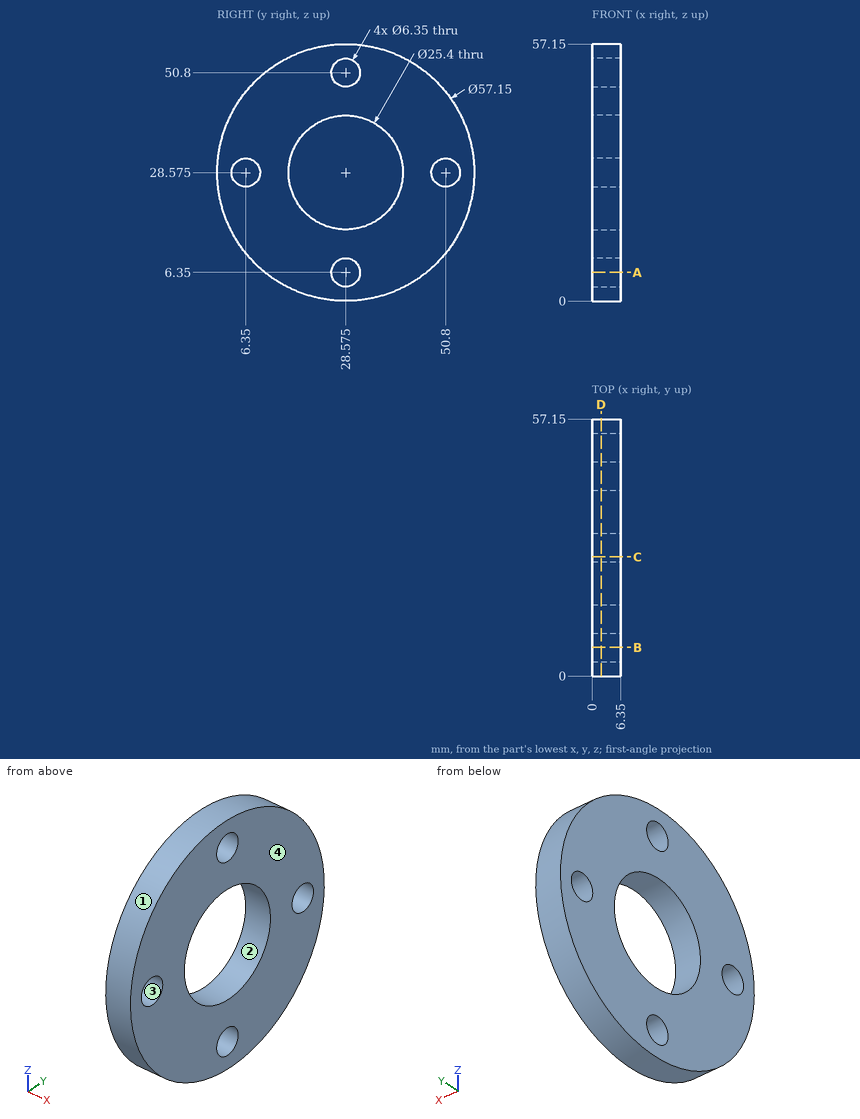
The drawing under review shows one solid part. Ordinate dimensions are in mm from its lowest x, y, z. Give positions to 0.01 mm unless a question says otherwise; leave off trailing zeros. Loops run counter-clockwise (first coordinate to the right, second up) from the corner with the lowest first, then second, coordinate; pieces in that order, holes last. Notation, with made-up numbers: M 0,26 L 24,26 A6 ccw 24,31 Z; hole C 60.5,3.5 d4. An arc over 180 degrees is marked long. One line per item, written item: value. Start each with the question number.
Q1. Add section A-A (z = 6.35). Give the boundary of the cut face in (x, y).
Q2. Draft analysis for pull direction Z (two halves, no side actions). For the marked faces 1, 2, 3 and 4, state which applies: released by +Z, released by -Z, zero draft, split by the parting line, or undercut.
Q3. Add section C-C (y = 26.5). Give the boundary of the cut face in (x, z), and give its area (3 significant figures).
Q4. Add section D-D (x = 2). Give the boundary of the cut face in (y, z) (3 decimals).
Q5. Clearance check with a flat-ended pin moving along its axis: pin 1 Ø3 at (x, y) = (3, 38.5) entering from -Z. State where the tip first meets the part, or that it passes through.
Q6. For L1, parallel to Z at x = 3.5, y = 27; L2, parallel to Y at x = 1, z = 31; L3, parallel to Z at x = 0.5, y = 34, list the stretches that pass through material, from the lowest coordinate up.
Reply:
1. outline: M 0,10.61 L 6.35,10.61 L 6.35,25.4 L 0,25.4 Z; M 0,31.75 L 6.35,31.75 L 6.35,46.54 L 0,46.54 Z
2. face 1: split by the parting line
2. face 2: undercut
2. face 3: undercut
2. face 4: zero draft
3. outline: M 0,0.08 L 6.35,0.08 L 6.35,3.95 L 0,3.95 Z; M 0,8.75 L 6.35,8.75 L 6.35,16.05 L 0,16.05 Z; M 0,41.1 L 6.35,41.1 L 6.35,48.4 L 0,48.4 Z; M 0,53.2 L 6.35,53.2 L 6.35,57.07 L 0,57.07 Z
3. area: 142 mm²
4. outline: C 28.575,28.575 d57.15; hole C 6.35,28.575 d6.35; hole C 28.575,28.575 d25.4; hole C 28.575,6.35 d6.35; hole C 28.575,50.8 d6.35; hole C 50.8,28.575 d6.35
5. pin 1: z = 1.27
6. L1: 0.04 to 3.59, 9.11 to 15.97, 41.18 to 48.04, 53.56 to 57.11
6. L2: 0.1 to 4.3, 8.4 to 16.11, 41.04 to 48.75, 52.85 to 57.05
6. L3: 0.52 to 17.09, 40.06 to 56.63
